```python
from build123d import *

# Parameters (mm, degrees)
F0_W     = 30
F0_H     = 10
F0_H_2   = 15
F1_DEPTH = 0.6
F2_W     = 30
F2_H     = 3
F3_DEPTH = 8
F5_DEPTH = 10
F7_DEPTH = 4


with BuildPart() as f1:
    # F0 (on Top) → F1 (new body)
    with BuildSketch(Plane.XY):
        with Locations((-15, 20)):
            Rectangle(F0_W, F0_H)
        with Locations((-15, 7.5)):
            Rectangle(F0_W, F0_H_2)
    extrude(amount=F1_DEPTH)

    # F2 (on face) → F3 (join)
    with BuildSketch(Plane.XY.offset(0.6)):
        with Locations((-15, 13.5)):
            Rectangle(F2_W, F2_H)
        with Locations((-15, 1.5)):
            Rectangle(F2_W, F2_H)
    extrude(amount=F3_DEPTH)

    # F4 (on face) → F5 (join)
    with BuildSketch(Plane(origin=(0, 15, 0), x_dir=(-1, 0, 0), z_dir=(0, 1, 0))):
        Polygon((24, 0.6), (0, 4.4), (0, 0.6), align=None)
    extrude(amount=F5_DEPTH)

    # F6 (on face) → F7 (join)
    with BuildSketch(Plane.XY.offset(0.6)):
        Polygon((-21.7479817708, 2.95), (-19.3169704861, 2.95), (-19.3169704861, 3), (-21.7767433449, 3), align=None)
        with BuildLine():
            Line((-17.0459201389, 11.9729817708), (-17.0459201389, 3))
            Line((-17.0459201389, 3), (-13.5546069033, 3))
            add(Edge.make_bspline(
                [(-10.8281792535, 4.1348958333), (-11.8363616657, 3.1934025301), (-13.5546069033, 3)],
                knots=[0, 0, 0, 0.7945789636, 0.7945789636, 0.7945789636], degree=2))
            add(Edge.make_bspline(
                [(-9.5593532986, 7.5473958333), (-9.5593532986, 5.3197916667), (-10.8281792535, 4.1348958333)],
                knots=[0, 0, 0, 1, 1, 1], degree=2))
            add(Edge.make_bspline(
                [(-10.7817708333, 10.8068467882), (-9.5593532986, 9.6407118056), (-9.5593532986, 7.5473958333)],
                knots=[0, 0, 0, 1, 1, 1], degree=2))
            add(Edge.make_bspline(
                [(-14.2140190972, 11.9729817708), (-12.0041883681, 11.9729817708), (-10.7817708333, 10.8068467882)],
                knots=[0, 0, 0, 1, 1, 1], degree=2))
            Line((-14.2140190972, 11.9729817708), (-17.0459201389, 11.9729817708))
        make_face()
        with BuildLine():
            add(Edge.make_bspline(
                [(-11.5480034722, 7.4980251736), (-11.5480034722, 10.4049696181), (-14.1152777778, 10.4049696181)],
                knots=[0, 0, 0, 1, 1, 1], degree=2))
            add(Edge.make_bspline(
                [(-14.3127604167, 4.5298611111), (-11.5480034722, 4.5298611111), (-11.5480034722, 7.4980251736)],
                knots=[0, 0, 0, 1, 1, 1], degree=2))
            Line((-14.3127604167, 4.5298611111), (-15.1323133681, 4.5298611111))
            Line((-15.1323133681, 4.5298611111), (-15.1323133681, 10.4049696181))
            Line((-15.1323133681, 10.4049696181), (-14.1152777778, 10.4049696181))
        make_face(mode=Mode.SUBTRACT)
        with BuildLine():
            add(Edge.make_bspline(
                [(-7.2167314747, 3), (-7.7620891499, 3.1339116551), (-8.2441189236, 3.3706380208)],
                knots=[0.5656812019, 0.5656812019, 0.5656812019, 1, 1, 1], degree=2))
            Line((-7.2167314747, 3), (-4.2997672598, 3))
            add(Edge.make_bspline(
                [(-3.2428710938, 3.5296115451), (-3.6847580589, 3.176002784), (-4.2997672598, 3)],
                knots=[0, 0, 0, 0.5022669023, 0.5022669023, 0.5022669023], degree=2))
            add(Edge.make_bspline(
                [(-2.3630859375, 5.4560546875), (-2.3630859375, 4.2336371528), (-3.2428710938, 3.5296115451)],
                knots=[0, 0, 0, 1, 1, 1], degree=2))
            add(Edge.make_bspline(
                [(-2.8321072049, 6.9460611979), (-2.3630859375, 6.3388020833), (-2.3630859375, 5.4560546875)],
                knots=[0, 0, 0, 1, 1, 1], degree=2))
            add(Edge.make_bspline(
                [(-4.5669921875, 8.1595920139), (-3.3011284722, 7.5533203125), (-2.8321072049, 6.9460611979)],
                knots=[0, 0, 0, 1, 1, 1], degree=2))
            add(Edge.make_bspline(
                [(-5.7785481771, 8.7915364583), (-5.5228081597, 8.6157769097), (-4.5669921875, 8.1595920139)],
                knots=[0, 0, 0, 1, 1, 1], degree=2))
            add(Edge.make_bspline(
                [(-6.1517903646, 9.1558919271), (-6.0342881944, 8.9672960069), (-5.7785481771, 8.7915364583)],
                knots=[0, 0, 0, 1, 1, 1], degree=2))
            add(Edge.make_bspline(
                [(-6.2692925347, 9.597265625), (-6.2692925347, 9.3444878472), (-6.1517903646, 9.1558919271)],
                knots=[0, 0, 0, 1, 1, 1], degree=2))
            add(Edge.make_bspline(
                [(-5.9789930556, 10.2568576389), (-6.2692925347, 10.0040798611), (-6.2692925347, 9.597265625)],
                knots=[0, 0, 0, 1, 1, 1], degree=2))
            add(Edge.make_bspline(
                [(-5.1456163194, 10.5096354167), (-5.6886935764, 10.5096354167), (-5.9789930556, 10.2568576389)],
                knots=[0, 0, 0, 1, 1, 1], degree=2))
            add(Edge.make_bspline(
                [(-4.2174479167, 10.3921332465), (-4.6894314236, 10.5096354167), (-5.1456163194, 10.5096354167)],
                knots=[0, 0, 0, 1, 1, 1], degree=2))
            add(Edge.make_bspline(
                [(-3.0226779514, 9.9784071181), (-3.7454644097, 10.2746310764), (-4.2174479167, 10.3921332465)],
                knots=[0, 0, 0, 1, 1, 1], degree=2))
            Line((-3.0226779514, 9.9784071181), (-2.4065321181, 11.4674262153))
            add(Edge.make_bspline(
                [(-3.7425021701, 11.9354600694), (-3.1036458333, 11.7695746528), (-2.4065321181, 11.4674262153)],
                knots=[0, 0, 0, 1, 1, 1], degree=2))
            add(Edge.make_bspline(
                [(-4.024584157, 12), (-3.8820128143, 11.971685399), (-3.7425021701, 11.9354600694)],
                knots=[0.781624387, 0.781624387, 0.781624387, 1, 1, 1], degree=2))
            Line((-4.024584157, 12), (-6.0945606148, 12))
            add(Edge.make_bspline(
                [(-7.3277994792, 11.4170681424), (-6.8285068793, 11.8380046043), (-6.0945606148, 12)],
                knots=[0, 0, 0, 0.6151547553, 0.6151547553, 0.6151547553], degree=2))
            add(Edge.make_bspline(
                [(-8.139453125, 9.5340711806), (-8.139453125, 10.7327907986), (-7.3277994792, 11.4170681424)],
                knots=[0, 0, 0, 1, 1, 1], degree=2))
            add(Edge.make_bspline(
                [(-7.8925998264, 8.42421875), (-8.139453125, 8.9001519097), (-8.139453125, 9.5340711806)],
                knots=[0, 0, 0, 1, 1, 1], degree=2))
            add(Edge.make_bspline(
                [(-7.2320203993, 7.5908420139), (-7.6457465278, 7.9482855903), (-7.8925998264, 8.42421875)],
                knots=[0, 0, 0, 1, 1, 1], degree=2))
            add(Edge.make_bspline(
                [(-5.9928168403, 6.8443576389), (-6.8182942708, 7.2333984375), (-7.2320203993, 7.5908420139)],
                knots=[0, 0, 0, 1, 1, 1], degree=2))
            add(Edge.make_bspline(
                [(-4.8227322049, 6.2331488715), (-5.1100694444, 6.4237196181), (-5.9928168403, 6.8443576389)],
                knots=[0, 0, 0, 1, 1, 1], degree=2))
            add(Edge.make_bspline(
                [(-4.3872829861, 5.8352213542), (-4.5353949653, 6.042578125), (-4.8227322049, 6.2331488715)],
                knots=[0, 0, 0, 1, 1, 1], degree=2))
            add(Edge.make_bspline(
                [(-4.2391710069, 5.3632378472), (-4.2391710069, 5.6278645833), (-4.3872829861, 5.8352213542)],
                knots=[0, 0, 0, 1, 1, 1], degree=2))
            add(Edge.make_bspline(
                [(-4.5758789063, 4.6473632812), (-4.2391710069, 4.8873046875), (-4.2391710069, 5.3632378472)],
                knots=[0, 0, 0, 1, 1, 1], degree=2))
            add(Edge.make_bspline(
                [(-5.5405815972, 4.407421875), (-4.9125868056, 4.407421875), (-4.5758789063, 4.6473632812)],
                knots=[0, 0, 0, 1, 1, 1], degree=2))
            add(Edge.make_bspline(
                [(-6.6988172743, 4.5733072917), (-6.0658854167, 4.407421875), (-5.5405815972, 4.407421875)],
                knots=[0, 0, 0, 1, 1, 1], degree=2))
            add(Edge.make_bspline(
                [(-8.2441189236, 5.1479817708), (-7.3317491319, 4.7391927083), (-6.6988172743, 4.5733072917)],
                knots=[0, 0, 0, 1, 1, 1], degree=2))
            Line((-8.2441189236, 5.1479817708), (-8.2441189236, 3.3706380208))
        make_face()
        with BuildLine():
            Line((-21.7767433449, 3), (-19.3169704861, 3))
            Line((-19.3169704861, 3), (-19.3169704861, 11.9729817708))
            Line((-19.3169704861, 11.9729817708), (-21.0390190972, 11.9729817708))
            Line((-21.0390190972, 11.9729817708), (-21.0390190972, 7.7014322917))
            add(Edge.make_bspline(
                [(-20.9462022569, 5.2151258681), (-21.0390190972, 6.9746961806), (-21.0390190972, 7.7014322917)],
                knots=[0, 0, 0, 1, 1, 1], degree=2))
            Line((-20.9462022569, 5.2151258681), (-20.9896484375, 5.2151258681))
            Line((-20.9896484375, 5.2151258681), (-24.9077039931, 11.9729817708))
            Line((-24.9077039931, 11.9729817708), (-27.3209418403, 11.9729817708))
            Line((-27.3209418403, 11.9729817708), (-27.3209418403, 3))
            Line((-27.3209418403, 3), (-25.6107421875, 3))
            Line((-25.6107421875, 3), (-25.6107421875, 7.1958767361))
            add(Edge.make_bspline(
                [(-25.7292317708, 9.775), (-25.6107421875, 7.9680338542), (-25.6107421875, 7.1958767361)],
                knots=[0, 0, 0, 1, 1, 1], degree=2))
            Line((-25.7292317708, 9.775), (-25.6739366319, 9.775))
            Line((-25.6739366319, 9.775), (-21.7767433449, 3))
        make_face()
    extrude(amount=F7_DEPTH)


solid = f1.part
```
Design review of the part built by this model. Coordinates are the model's own, in mm. A direction names the side the tool comes from. Round coordinates to 2 decimals unless told otherwise and drop trailing zeros. Order: outer loops, then holes, each group sorted by start corner. A loop starts at its lowest first (then second) coordinate and runs counter-clockwise, first axis right, second up. Notation, with made-up numbers: (18, 5) - (36, 5) arc R9 ccw to (36, 11) - close; hole circle Ø1 at (83.5, -33.5). An arc over 180 degrees is marked (long way). Return JSON: item names as keys, results as strings.
Q1. Consider section B-B on y = 18. Write out the cut boundary in (x, z), plus the area to 3 significant figures.
Computed values:
{"outline": "(-30, 0) - (0, 0) - (0, 4.4) - (-24, 0.6) - (-30, 0.6) - close", "area": "63.6 mm2"}
Q2. Consider section A-A on z = 6.25. Write out the cut boundary in (x, y).
Computed values:
{"outline": "(-30, 0) - (0, 0) - (0, 3) - (-30, 3) - close; (-30, 12) - (0, 12) - (0, 15) - (-30, 15) - close"}
Q3. The part is to be moulded in two halves that separate along X. For faces 4 (the flat face through (-15, 14, 8.6)), 5 (the flat face through (-15.132, 7, 3)), say which applies: pulls with the +X half, pulls with the -X half, needs draft (parallel to the pull), parting line crosses it, or undercut.
Computed values:
{"face 4": "needs draft", "face 5": "undercut"}
Q4. Wall thickness on L1, parallel to X at y = 5, z = 3.75; L2, parallel to Y at x = -12.5, z = 2; L3, parallel to X at y = 3.75, z = 1: over which ranges is each line inside the solid? List them lowest first. Write a range as [from, to].
Computed values:
{"L1": "x = [-27.32, -25.61], [-22.93, -19.32], [-17.05, -15.13], [-12.55, -10.15], [-8.24, -7.9], [-4.3, -2.4]", "L2": "y = [0, 3], [3.21, 5.04], [9.96, 11.76], [12, 25]", "L3": "x = [-27.32, -25.61], [-22.21, -19.32], [-17.05, -11.32], [-8.24, -3]"}
Q5. For pin 1 Ø1.2 at (y, z) = (9.5, 2.5) entering from -X; pin 2 Ø2 at (y, z) = (7, 2) entering from +X; pin 3 Ø4.5 at (x, y) = (-6, 6.5) entering from +Z, all flat-tipped, find the tip position at first contact; note any pin that passes through.
Computed values:
{"pin 1": "stops at x = -27.32", "pin 2": "stops at x = -2.41", "pin 3": "stops at z = 4.6"}
Q6. Machinability: for faces 1 (the flat face through (-23, 8, 4.6)), 2 (the flat face through (-15, 15, 5)), 3 (the flat face through (-14.7, 4.53, 2.6)), which of the approach directions +Z, -Z, +X, -X, +Y, -Y give a long, thin tool a straight path to every point of the face, cutting with its end or side? Answer none if there is none.
Computed values:
{"face 1": "+Z, +X, -X", "face 2": "+Z, -X, +Y", "face 3": "+Z"}
Q7. Consider section D-D on z = 2.5. Give the number of separate pieces and of enclosed holes in the cut face, plus the area to 3 significant figures.
Computed values:
{"separate pieces": "1", "enclosed holes": "2", "area": "417 mm2"}
